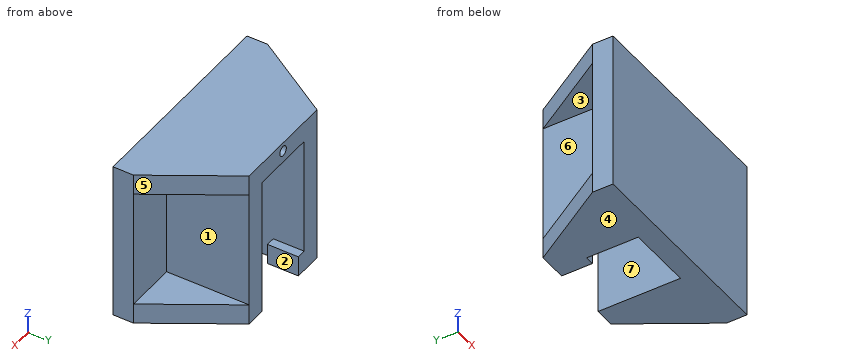
Autodesk Inventor part; units mm, degrees
ref_plane "YZ Plane" through (0, 0, 0) normal (1, 0, 0) x (0, 1, 0)
ref_plane "XZ Plane" through (0, 0, 0) normal (0, 1, 0) x (-1, 0, 0)
ref_plane "XY Plane" through (0, 0, 0) normal (0, 0, 1) x (1, 0, 0)
sketch "Sketch1" plane through (0, 0, 0) normal (0, 1, 0) x (-1, 0, 0)
  point P0 (0, 0)
sketch "Sketch2" plane through (0, 0, 0) normal (0, 1, 0) x (-1, 0, 0)
  line L0 (-10.25, -15.5) -> (10.25, -15.5)
  line L1 (10.25, -15.5) -> (10.25, 15.5)
  line L2 (10.25, 15.5) -> (-10.25, 15.5)
  line L3 (-10.25, 15.5) -> (-10.25, -15.5)
  line L4 (-10.25, -15.5) -> (10.25, 15.5) construction
  line L5 (10.25, -15.5) -> (-10.25, 15.5) construction
  point P0 (0, 0)
  dimension "d0" = 20.5
  dimension "d1" = 31
extrude "Extrusion1" add sketch "Sketch2" along normal blind 20
sketch "Sketch3" plane through (0, 20, 0) normal (0, 1, 0) x (1, 0, 0)
  line L0 (6.375, -11.5) -> (-6.375, -11.5)
  line L1 (-6.375, -11.5) -> (-6.375, 11.5)
  line L2 (-6.375, 11.5) -> (6.375, 11.5)
  line L3 (6.375, 11.5) -> (6.375, -11.5)
  line L4 (10.25, 15.5) -> (-10.25, 15.5)
  line L5 (10.25, -15.5) -> (10.25, 15.5)
  line L6 (-10.25, 15.5) -> (-10.25, -15.5)
  line L7 (-10.25, -15.5) -> (10.25, -15.5)
  point P0 (0, 0)
  dimension "d4" = 23
  dimension "d5" = 12.75
  dimension "d6" = 4
  dimension "d7" = 3.875
  dimension "d8" = 3.875
  dimension "d9" = 4
extrude "Extrusion2" cut sketch "Sketch3" against normal blind 16 contours L0 L1 L2 L3
sketch "Sketch4" plane through (10.25, 0, -15.5) normal (0, 0, -1) x (-1, 0, 0)
  line L0 (16.625, 14) -> (3.875, 14)
  line L1 (3.875, 14) -> (3.875, 4)
  line L2 (3.875, 4) -> (16.625, 4)
  line L3 (16.625, 4) -> (16.625, 14)
  line L4 (3.875, 20) -> (16.625, 20)
  line L5 (0, 0) -> (20.5, 0)
  line L6 (0, 0) -> (0, 20)
  line L7 (20.5, 0) -> (20.5, 20)
  point P0 (10.25, 0)
  dimension "d12" = 10
  dimension "d13" = 12.75
  dimension "d14" = 4
  dimension "d15" = 3.875
  dimension "d16" = 3.875
  dimension "d17" = 6
extrude "Extrusion3" cut sketch "Sketch4" against normal blind 4
sketch "Sketch5" plane through (0, 20, 0) normal (0, 1, 0) x (1, 0, 0)
  circle A0 centre (0, -13.8) radius 0.975
  line L0 (6.375, -11.5) -> (-6.375, -11.5)
  line L1 (10.25, -15.5) -> (10.25, 15.5)
  line L2 (-10.25, 15.5) -> (-10.25, -15.5)
  circle A1 centre (0, 13.8) radius 0.975
  line L3 (-6.375, 11.5) -> (6.375, 11.5)
  point P0 (0, 0)
  dimension "d20" = 1.95
  dimension "d21" = 2.3
  dimension "d22" = 10.25
  dimension "d23" = 10.25
  dimension "d24" = 1.95
  dimension "d25" = 2.3
  dimension "d26" = 10.25
  dimension "d27" = 10.25
extrude "Extrusion4" cut sketch "Sketch5" against normal blind 8
sketch "Sketch6" plane through (-10.25, 0, -15.5) normal (-1, 0, 0) x (0, 0, 1)
  line L0 (0, 4) -> (27, 4)
  line L1 (0, 0) -> (31, 0)
  line L2 (0, 4) -> (31, 4)
  line L3 (31, 4) -> (31, 0)
  line L4 (31, 0) -> (0, 0)
  line L5 (0, 0) -> (0, 4)
  point P0 (15.5, 0)
extrude "Extrusion5" add sketch "Sketch6" along normal blind 10
sketch "Sketch8" plane through (10.25, 0, 15.5) normal (1, 0, 0) x (0, 0, -1)
  line L0 (31, 4) -> (4, 4)
  line L1 (0, 0) -> (31, 0)
  line L2 (31, 4) -> (0, 4)
  line L3 (0, 4) -> (0, 0)
  line L4 (0, 0) -> (31, 0)
  line L5 (31, 0) -> (31, 4)
  point P0 (15.5, 0)
  point P1 (4, 4)
extrude "Extrusion6" add sketch "Sketch8" along normal blind 10
sketch "Sketch9" plane through (10.25, 20, -15.5) normal (0, 0, -1) x (-1, 0, 0)
  line L0 (20.5, -16) -> (20.5, 0)
  line L1 (20.5, 0) -> (20.5, -16)
  line L2 (30.5, -20) -> (30.5, -16)
  line L3 (20.5, -16) -> (30.5, -16)
  line L4 (30.5, -16) -> (20.5, 0)
  line L5 (0, -16) -> (0, 0)
  line L6 (0, 0) -> (0, -16)
  line L7 (0, -16) -> (-10, -16)
  line L8 (0, -16) -> (-10, -16)
  line L9 (-10, -16) -> (0, 0)
  point P0 (10.25, -20)
extrude "Extrusion7" add sketch "Sketch9" against normal blind 4
sketch "Sketch10" plane through (-10.25, 20, 15.5) normal (0, 0, 1) x (1, 0, 0)
  line L0 (0, 0) -> (0, -16)
  line L1 (0, -16) -> (-10, -16)
  line L2 (0, -16) -> (-10, -16)
  line L3 (-10, -16) -> (0, 0)
  line L4 (-10, -16) -> (0, 0)
  line L5 (20.5, -16) -> (20.5, 0)
  line L6 (20.5, 0) -> (20.5, -16)
  line L7 (20.5, -16) -> (30.5, -16)
  line L8 (20.5, -16) -> (30.5, -16)
  line L9 (30.5, -16) -> (20.5, 0)
  point P0 (10.25, -20)
extrude "Extrusion8" add sketch "Sketch10" against normal blind 4
sketch "Sketch11" plane through (0, 20, 0) normal (0, 1, 0) x (1, 0, 0)
  line L0 (6.375, 15.5) -> (6.375, -11.5)
  line L1 (-6.375, 11.5) -> (6.375, 11.5)
  line L2 (6.375, 15.5) -> (-4.625, 15.5)
  line L3 (-4.625, 15.5) -> (-4.625, 11.5)
  line L4 (-4.625, 11.5) -> (6.375, 11.5)
  line L5 (6.375, 11.5) -> (6.375, 15.5)
  point P0 (0, 0)
  dimension "d38" = 11
extrude "Extrusion9" cut sketch "Sketch11" against normal blind 6
properties part number "servommount1"
Verification items for the finished model (mm, model axes). Face numbers are marked on the shaded views. A direction names the side the tool comes from. Coordinates: 2 decimals unless noted, no trailing zeros. Write each loop counter-clockwise with the first axis right and the second up, starting at its lowest first coordinate (ties: lowest second). Pieces come first, ordered by that corner, then holes. Notation, with made-up numbers: (-18.75, 62) -> (31.25, 62) arc R18 ccw to (31.25, 86) -> close; hole circle Ø7 at (-23.5, 4.25). An arc over 180 degrees is marked (long way). One line per item, written item: value. Start each with the question number.
Q1. Go/stop test with flat-tipped pins: P1, Ø8, axis at x = 17.5, z = 5.5, coming from the +Y side; P2, Ø2, axis at y = 16, z = -14.5, coming from the +X side (3 decimals); P3, Ø3, axis at y = 10, z = -11.5, coming from the +X side. Record where each tip stops, or that it passes through.
Q2. Cross-section at A-A on x = -5.5. Enter the section's corners in (y, z).
Q3. Cross-section at B-B on z = -4.5. Enter the section's corners in (x, y) (3 decimals).
Q4. Cross-section at D-D on y = 19. Enter the section's corners in (x, z) (3 decimals).
Q5. Mould release check, pull along X, two halves, no side actions. Record for the marked faces 4, 5, 6 and 7: pulls with the +X half, pulls with the -X half, needs draft (parallel to the pull), parting line crosses it, or undercut.
Q6. Thickness scan on L1, parallel to X at y = 10.25, z = -10 (3 decimals); L2, parallel to Z at x = 0, y = 17 (3 decimals); L3, parallel to Z at x = -2, y = 7.25. Record the ranges inside material, lowest first. Write a range as from..to.
Q7. Access from +Z, -Z, +X, -X, +Y, -Y to the whole of each face (thin tool, end or side, straight path). Record for the marked faces 1, 2 and 3.
Q8. Cross-section at C-C on x = 13. Enter the section's corners in (y, z).
Checked values:
1. P1: stops at y = 4
1. P2: stops at x = 13.375
1. P3: stops at x = 17.44
2. outline: (0, -15.5) -> (4, -15.5) -> (4, 11.5) -> (20, 11.5) -> (20, 15.5) -> (0, 15.5) -> close; (14, -15.5) -> (20, -15.5) -> (20, -11.5) -> (14, -11.5) -> close
3. outline: (-20.25, 0) -> (20.25, 0) -> (20.25, 4) -> (10.25, 4) -> (10.25, 20) -> (6.375, 20) -> (6.375, 4) -> (-6.375, 4) -> (-6.375, 20) -> (-10.25, 20) -> (-10.25, 4) -> (-20.25, 4) -> close
4. outline: (-10.875, -15.5) -> (-4.625, -15.5) -> (-4.625, -11.5) -> (-6.375, -11.5) -> (-6.375, 11.5) -> (6.375, 11.5) -> (6.375, -15.5) -> (10.875, -15.5) -> (10.875, -11.5) -> (10.25, -11.5) -> (10.25, 11.5) -> (10.875, 11.5) -> (10.875, 15.5) -> (-10.875, 15.5) -> (-10.875, 11.5) -> (-10.25, 11.5) -> (-10.25, -11.5) -> (-10.875, -11.5) -> close; hole circle Ø1.95 at (0, 13.8)
5. face 4: needs draft
5. face 5: pulls with the +X half
5. face 6: pulls with the -X half
5. face 7: undercut
6. L1: x = -10.25..-6.375, 6.375..10.25
6. L2: z = 11.5..12.825, 14.775..15.5
6. L3: z = 11.5..15.5
7. face 1: +X, +Y
7. face 2: -Z, +Y
7. face 3: -X, +Y
8. outline: (0, -15.5) -> (15.6, -15.5) -> (15.6, -11.5) -> (4, -11.5) -> (4, 11.5) -> (15.6, 11.5) -> (15.6, 15.5) -> (0, 15.5) -> close
